Geometry: final body of the model. Coordinates: model frame, mm. Give positions to 0.01 mm unless a question says otherwise; leave off trailing zeros. Loops run counter-clockwise (first coordinate to the right, second up) from the corner with the lowest first, then second, coordinate; pieces in that order, holes last. Notation, with made-up numbers: (42.5, 88) - (63.5, 88) arc R13 ccw to (63.5, 103) - close; hole circle Ø3 at (76, 47). An arc over 180 degrees is marked (long way). Answer in a Markdown table with one row per item.
from build123d import *

# Parameters (mm, degrees)
F0_W     = 736.6
F0_H     = 304.8
F1_DEPTH = 19.05
F2_W     = 12.7
F2_H     = 12.7
F3_DEPTH = 736.601
F4_W     = 12.7
F4_H     = 12.7
F5_DEPTH = 304.801


with BuildPart() as f1:
    # F0 (on Front) → F1 (new body)
    with BuildSketch(Plane.XZ):
        with Locations((368.3, 152.4)):
            Rectangle(F0_W, F0_H)
    extrude(amount=F1_DEPTH)

    # F2 (on face) → F3 (cut, through all)
    with BuildSketch(Plane.YZ.offset(736.6)):
        with Locations((-12.7, 6.35)):
            Rectangle(F2_W, F2_H)
    extrude(amount=-F3_DEPTH, mode=Mode.SUBTRACT)

    # F4 (on face) → F5 (cut, through all)
    with BuildSketch(Plane.XY.offset(304.8)):
        with Locations((6.35, -12.7)):
            Rectangle(F4_W, F4_H)
    extrude(amount=-F5_DEPTH, mode=Mode.SUBTRACT)


solid = f1.part
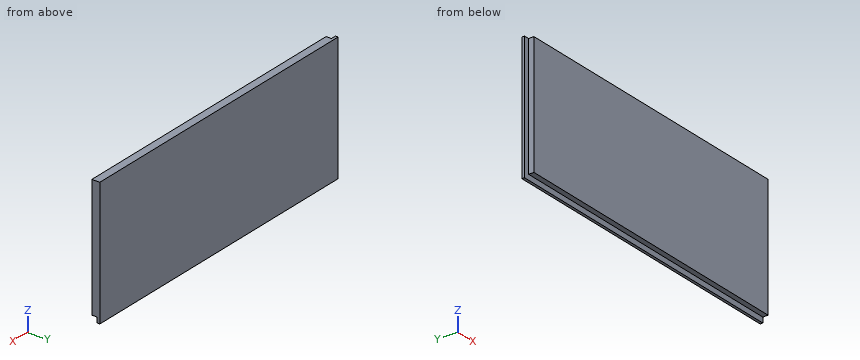
Q1. Cut plane A-A (x = 439.5). Output: boundary loops of the cut face in (y, z).
Check values:
| item | result |
|---|---|
| outline | (-19.05, 12.7) - (-6.35, 12.7) - (-6.35, 0) - (0, 0) - (0, 304.8) - (-19.05, 304.8) - close |
Q2. Cut plane B-B (y = -14.75). Output: boundary loops of the cut face in (x, z), and give its area (3 significant figures).
Check values:
| item | result |
|---|---|
| outline | (12.7, 12.7) - (736.6, 12.7) - (736.6, 304.8) - (12.7, 304.8) - close |
| area | 211,000 mm² |
Q3. Material intervals for line 1 along Z through (x, y) = (206.5, -10.5); line 2 along X through (y, z) = (-12, 86), sorted ascending.
Check values:
| item | result |
|---|---|
| line 1 | 12.7 to 304.8 |
| line 2 | 12.7 to 736.6 |
Q4. First-contact query: pin 1 (3 mm diameter, centred on x = 146, z = 273.5, fed in from +Y); pin 2 (8 mm diameter, centred on x = 281.5, y = -12.5, fed in from -Z); pin 3 (6.5 mm diameter, centred on y = -11, z = 100.5, fed in from -X). Flat tips, straight axial feed; report the tip coordinate or a pass-through.
Check values:
| item | result |
|---|---|
| pin 1 | y = 0 |
| pin 2 | z = 12.7 |
| pin 3 | x = 12.7 |
